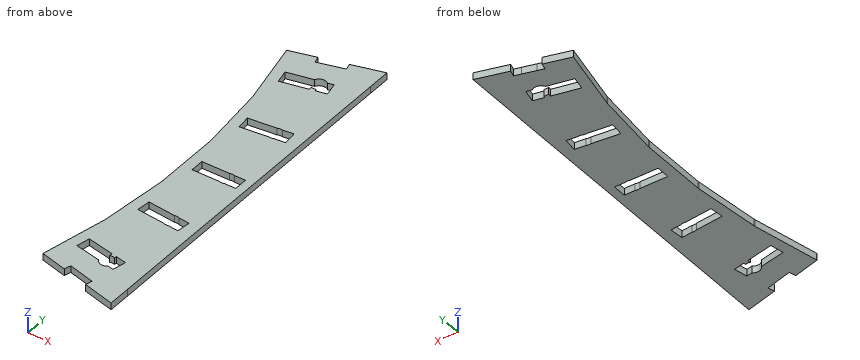
Autodesk Inventor part; units mm, degrees
ref_plane "Work Plane2" through (388.0538, -686.9281, 216.8066) normal (0, 0, 1) x (-0.9917, -0.1283, 0)
ref_plane "YZ Plane" through (0, 0, 0) normal (1, 0, 0) x (0, 1, 0)
ref_plane "XZ Plane" through (0, 0, 0) normal (0, 1, 0) x (-1, 0, 0)
ref_plane "Work Plane2" through (388.0538, -686.9281, 216.8066) normal (0, 0, 1) x (-0.9917, -0.1283, 0)
sketch "Sketch3" plane through (388.0538, -686.9281, 216.8066) normal (0, 0, 1) x (-0.9917, -0.1283, 0)
  line L0 (4.3583, 15.8159) -> (10.8533, 46.3726) construction
  line L1 (1.0044, -15.8113) -> (4.2698, 15.2569) construction
  line L2 (1.0044, -15.8113) -> (4.2698, 15.2569) construction
  line L3 (0.9748, -47.6157) -> (0.9748, -16.3764) construction
  line L4 (0.9748, -47.6157) -> (0.9748, -16.3764) construction
  line L5 (4.2698, -79.2491) -> (1.0044, -48.1809) construction
  line L6 (4.2698, -79.2491) -> (1.0044, -48.1809) construction
  line L7 (10.9998, 46.9192) -> (20.6533, 76.6296) construction
  line L8 (4.3583, 15.8159) -> (10.8533, 46.3726) construction
  line L9 (10.9998, 46.9192) -> (20.6533, 76.6296) construction
  line L10 (20.6533, 76.6296) -> (-103.8397, 124.4179) construction
  line L11 (-117.8064, 81.4327) -> (10.9998, 46.9192) construction
  line L12 (10.8533, 46.3726) -> (-117.9529, 80.8861) construction
  line L13 (-127.3499, 36.6764) -> (4.3583, 15.8159) construction
  line L14 (4.2698, 15.2569) -> (-127.4385, 36.1175) construction
  line L15 (0.9748, -16.3764) -> (-132.1925, -9.3974) construction
  line L16 (-132.1629, -8.8323) -> (1.0044, -15.8113) construction
  line L17 (1.0044, -48.1809) -> (-132.1629, -55.1599) construction
  line L18 (-132.1925, -54.5947) -> (0.9748, -47.6157) construction
  line L19 (-127.4385, -100.1096) -> (4.2698, -79.2491) construction
  line L20 (19.0965, 77.2271) -> (9.3891, 47.3508)
  line L21 (9.3891, 47.3508) -> (9.2426, 46.8041)
  line L22 (9.2426, 46.8041) -> (2.7113, 16.0767)
  line L23 (2.7113, 16.0767) -> (2.6228, 15.5178)
  line L24 (2.6228, 15.5178) -> (-0.6609, -15.724)
  line L25 (-0.6609, -15.724) -> (-0.6905, -16.2891)
  line L26 (-0.6905, -16.2891) -> (-0.6905, -47.703)
  line L27 (-0.6905, -47.703) -> (-0.6609, -48.2681)
  line L28 (-0.6609, -48.2681) -> (2.6228, -79.5099)
  line L29 (2.6228, -79.5099) -> (-36.3059, -75.4184)
  line L30 (-36.3059, -75.4184) -> (-19.8322, 81.3187)
  line L31 (-19.8322, 81.3187) -> (19.0965, 77.2271)
  line L32 (-127.4385, 36.1175) -> (-129.1369, 19.9578) construction
  point P0 (296.7492, -731.0239)
  dimension "d32" = 1.6652
  dimension "d33" = 1.6652
  dimension "d34" = 1.6652
  dimension "d35" = 1.6652
  dimension "d36" = 1.6652
  dimension "d37" = 29.21
extrude "Extrusion3" add sketch "Sketch3" along normal blind 3.175
sketch "Sketch5" plane through (388.0538, -686.9281, 219.9816) normal (0, 0, 1) x (0.9917, 0.1283, 0)
  line L0 (-19.0965, -77.2271) -> (19.8322, -81.3187)
  line L1 (-19.0965, -77.2271) -> (-19.1979, -77.4913)
  line L2 (-19.1979, -77.4913) -> (-7.3415, -82.0426)
  line L3 (4.515, -86.5938) -> (18.7052, -92.0409)
  line L4 (19.8322, -81.3187) -> (36.3059, 75.4184)
  line L5 (19.8322, -81.3187) -> (18.7052, -92.0409)
  line L6 (-18.0601, -74.5272) -> (-19.1979, -77.4913) construction
  line L7 (36.3059, 75.4184) -> (37.4328, 86.1406)
  line L8 (37.4328, 86.1406) -> (22.4202, 83.7628)
  line L9 (9.8766, 81.7761) -> (-2.6671, 79.7894)
  line L10 (36.3059, 75.4184) -> (-2.6228, 79.5099)
  line L11 (-2.6671, 79.7894) -> (-2.6228, 79.5099)
  line L12 (-2.6671, 79.7894) -> (-2.1704, 76.6535) construction
  line L13 (1.5509, -85.456) -> (-4.3773, -83.1804)
  line L14 (2.6887, -82.4919) -> (1.5509, -85.456)
  line L15 (-3.2395, -80.2163) -> (2.6887, -82.4919)
  line L16 (-3.2395, -80.2163) -> (-4.3773, -83.1804)
  line L17 (19.781, 80.1302) -> (13.5092, 79.1369)
  line L18 (19.2843, 83.2662) -> (19.781, 80.1302)
  line L19 (13.0125, 82.2728) -> (19.2843, 83.2662)
  line L20 (13.0125, 82.2728) -> (13.5092, 79.1369)
  line L21 (-4.3773, -83.1804) -> (-7.3415, -82.0426)
  line L22 (-3.2395, -80.2163) -> (-4.3773, -83.1804)
  line L23 (-6.2036, -79.0785) -> (-3.2395, -80.2163)
  line L24 (-7.3415, -82.0426) -> (-6.2036, -79.0785)
  line L25 (4.515, -86.5938) -> (1.5509, -85.456)
  line L26 (5.6528, -83.6297) -> (4.515, -86.5938)
  line L27 (2.6887, -82.4919) -> (5.6528, -83.6297)
  line L28 (2.6887, -82.4919) -> (1.5509, -85.456)
  line L29 (22.9169, 80.6269) -> (19.781, 80.1302)
  line L30 (22.4202, 83.7628) -> (22.9169, 80.6269)
  line L31 (19.2843, 83.2662) -> (22.4202, 83.7628)
  line L32 (19.2843, 83.2662) -> (19.781, 80.1302)
  line L33 (13.5092, 79.1369) -> (10.3733, 78.6402)
  line L34 (13.0125, 82.2728) -> (13.5092, 79.1369)
  line L35 (9.8766, 81.7761) -> (13.0125, 82.2728)
  line L36 (10.3733, 78.6402) -> (9.8766, 81.7761)
  point P0 (-296.7492, 731.0239)
  point P1 (19.781, 80.1302)
  point P2 (13.5092, 79.1369)
  point P3 (2.6887, -82.4919)
extrude "Extrusion4" add sketch "Sketch5" against normal blind 3.175 contours L10 L11 L9 L36 L33 L17 L29 L30 L8 L7 | L0 L5 L3 L26 L27 L15 L23 L24 L2 L1
sketch "Sketch6" plane through (388.0538, -686.9281, 219.9816) normal (0, 0, 1) x (0.9917, 0.1283, 0)
  line L0 (16.6451, 79.6336) -> (18.6318, 67.0899) construction
  line L1 (-0.2754, -81.3541) -> (4.2759, -69.4976) construction
  line L2 (18.7052, -92.0409) -> (37.4328, 86.1406) construction
  line L3 (28.069, -2.9502) -> (17.9647, -1.8882) construction
  line L4 (-6.2036, -79.0785) -> (5.6528, -83.6297) construction
  line L5 (22.9169, 80.6269) -> (10.3733, 78.6402) construction
  point P0 (-296.7492, 731.0239)
  dimension "d23" = 12.7
  dimension "d24" = 12.7
  dimension "d55" = 10.16
hole "Hole2" at (401.2076, -755.3034, 219.9816) at (397.9274, -618.0027, 219.9816) at (406.1123, -686.4967, 219.9816) direction (0, 0, -1) diameter 6.7564 depth 13.6144
sketch "Sketch7" plane through (388.0538, -686.9281, 219.9816) normal (0, 0, 1) x (0.9917, 0.1283, 0)
  line L0 (0.6609, 15.724) -> (-2.6228, -15.5178) construction
  line L1 (-0.981, 0.1031) -> (10.3864, -1.0917) construction
  line L2 (3.6239, -3.5734) -> (16.4852, -4.9251)
  line L3 (16.4852, -4.9251) -> (17.1489, 1.3901)
  line L4 (17.1489, 1.3901) -> (4.2877, 2.7418)
  line L5 (4.2877, 2.7418) -> (3.6239, -3.5734)
  line L6 (3.6239, -3.5734) -> (17.1489, 1.3901) construction
  line L7 (16.4852, -4.9251) -> (4.2877, 2.7418) construction
  circle A0 centre (17.9647, -1.8882) radius 3.3782 construction
  line L8 (10.8679, -38.2669) -> (-1.7816, -35.5781)
  line L9 (-1.7816, -35.5781) -> (-0.4614, -29.3669)
  line L10 (-0.4614, -29.3669) -> (12.1881, -32.0556)
  line L11 (12.1881, -32.0556) -> (10.8679, -38.2669)
  line L12 (10.8679, -38.2669) -> (-0.4614, -29.3669) construction
  line L13 (-1.7816, -35.5781) -> (12.1881, -32.0556) construction
  line L14 (-10.5029, -66.8425) -> (1.7962, -70.8387)
  line L15 (1.7962, -70.8387) -> (3.7585, -64.7995)
  line L16 (3.7585, -64.7995) -> (-8.5407, -60.8033)
  line L17 (-8.5407, -60.8033) -> (-10.5029, -66.8425)
  line L18 (-10.5029, -66.8425) -> (3.7585, -64.7995) construction
  line L19 (1.7962, -70.8387) -> (-8.5407, -60.8033) construction
  line L20 (18.5865, 35.1711) -> (5.6544, 35.1711)
  line L21 (5.6544, 35.1711) -> (5.6544, 28.8211)
  line L22 (5.6544, 28.8211) -> (18.5865, 28.8211)
  line L23 (18.5865, 28.8211) -> (18.5865, 35.1711)
  line L24 (18.5865, 35.1711) -> (5.6544, 28.8211) construction
  line L25 (5.6544, 35.1711) -> (18.5865, 28.8211) construction
  line L26 (3.6239, 67.5655) -> (4.2877, 61.2503)
  line L27 (4.2877, 61.2503) -> (17.1489, 62.6021)
  line L28 (17.1489, 62.6021) -> (16.4852, 68.9173)
  line L29 (16.4852, 68.9173) -> (3.6239, 67.5655)
  line L30 (3.6239, 67.5655) -> (17.1489, 62.6021) construction
  line L31 (4.2877, 61.2503) -> (16.4852, 68.9173) construction
  line L32 (-9.3891, -47.3508) -> (-19.0965, -77.2271) construction
  line L33 (-14.2428, -62.289) -> (-3.3722, -65.821) construction
  line L34 (-2.7113, -16.0767) -> (-9.2426, -46.8041) construction
  line L35 (-5.977, -31.4404) -> (5.2033, -33.8169) construction
  line L36 (0.6905, 47.703) -> (0.6905, 16.2891) construction
  line L37 (0.6905, 31.9961) -> (12.1205, 31.9961) construction
  line L38 (-2.6228, 79.5099) -> (0.6609, 48.2681) construction
  line L39 (-0.981, 63.889) -> (10.3864, 65.0838) construction
  line L40 (18.7804, -5.1664) -> (19.4442, 1.1488)
  line L41 (19.4442, 1.1488) -> (24.4964, 0.6178)
  line L42 (24.4964, 0.6178) -> (23.8326, -5.6974)
  line L43 (23.8326, -5.6974) -> (18.7804, -5.1664)
  line L44 (18.7804, -5.1664) -> (24.4964, 0.6178) construction
  line L45 (19.4442, 1.1488) -> (23.8326, -5.6974) construction
  line L46 (13.1254, -38.7467) -> (14.4456, -32.5355)
  line L47 (14.4456, -32.5355) -> (19.4146, -33.5916)
  line L48 (19.4146, -33.5916) -> (18.0943, -39.8029)
  line L49 (18.0943, -39.8029) -> (13.1254, -38.7467)
  line L50 (13.1254, -38.7467) -> (19.4146, -33.5916) construction
  line L51 (14.4456, -32.5355) -> (18.0943, -39.8029) construction
  line L52 (20.8944, 28.8211) -> (20.8944, 35.1711)
  line L53 (20.8944, 35.1711) -> (25.9744, 35.1711)
  line L54 (25.9744, 35.1711) -> (25.9744, 28.8211)
  line L55 (25.9744, 28.8211) -> (20.8944, 28.8211)
  line L56 (20.8944, 28.8211) -> (25.9744, 35.1711) construction
  line L57 (20.8944, 35.1711) -> (25.9744, 28.8211) construction
  line L58 (3.9912, -71.5519) -> (5.9534, -65.5127)
  line L59 (5.9534, -65.5127) -> (10.7848, -67.0825)
  line L60 (10.7848, -67.0825) -> (8.8225, -73.1217)
  line L61 (8.8225, -73.1217) -> (3.9912, -71.5519)
  line L62 (3.9912, -71.5519) -> (10.7848, -67.0825) construction
  line L63 (5.9534, -65.5127) -> (8.8225, -73.1217) construction
  line L64 (19.4442, 62.8433) -> (18.7804, 69.1585)
  line L65 (18.7804, 69.1585) -> (23.8326, 69.6895)
  line L66 (23.8326, 69.6895) -> (24.4964, 63.3743)
  line L67 (24.4964, 63.3743) -> (19.4442, 62.8433)
  line L68 (19.4442, 62.8433) -> (23.8326, 69.6895) construction
  line L69 (18.7804, 69.1585) -> (24.4964, 63.3743) construction
  point P0 (-296.7492, 731.0239)
  point P1 (5.2033, -33.8169)
  point P2 (-3.3722, -65.821)
  point P3 (12.1205, 31.9961)
  point P4 (10.3864, 65.0838)
  point P5 (21.6384, -2.2743)
  dimension "d38" = 11.43
  dimension "d39" = 6.35
  dimension "d40" = 12.9321
  dimension "d41" = 11.43
  dimension "d42" = 11.43
  dimension "d43" = 11.43
  dimension "d44" = 11.43
  dimension "d45" = 6.35
  dimension "d46" = 6.35
  dimension "d47" = 6.35
  dimension "d48" = 6.35
  dimension "d49" = 12.9321
  dimension "d50" = 12.9321
  dimension "d51" = 12.9321
  dimension "d52" = 12.9321
  dimension "d66" = 6.35
  dimension "d67" = 5.08
  dimension "d68" = 2.3079
  dimension "d69" = 6.35
  dimension "d70" = 5.08
  dimension "d71" = 6.35
  dimension "d72" = 5.08
  dimension "d73" = 6.35
  dimension "d74" = 5.08
  dimension "d75" = 6.35
  dimension "d76" = 5.08
  dimension "d77" = 2.3079
  dimension "d78" = 2.3079
  dimension "d79" = 2.3079
  dimension "d80" = 2.3079
extrude "Extrusion5" cut sketch "Sketch7" against normal blind 3.175
sketch "Sketch8" plane through (388.0538, -686.9281, 219.9816) normal (0, 0, 1) x (0.9917, 0.1283, 0)
  line L0 (0.6609, 15.724) -> (-2.6228, -15.5178) construction
  arc A0 (16.4852, -4.9251) -> (17.1489, 1.3901) centre (17.9647, -1.8882) ccw construction
  line L1 (18.5865, 35.1711) -> (18.5865, 28.8211) construction
  line L2 (18.5865, 31.9961) -> (19.7405, 31.9961) construction
  line L3 (0.6905, 47.703) -> (0.6905, 16.2891) construction
  line L4 (10.8679, -38.2669) -> (12.1881, -32.0556) construction
  line L5 (11.528, -35.1612) -> (12.6567, -35.4012) construction
  line L6 (-2.7113, -16.0767) -> (-9.2426, -46.8041) construction
  point P0 (-296.7492, 731.0239)
  point P1 (-0.6491, 3.2607)
  point P2 (0.6905, 35.1711)
  point P3 (-5.3169, -28.3348)
  dimension "d56" = 19.05
  dimension "d57" = 19.05
  dimension "d58" = 19.05
hole "Hole3" at (403.5277, -652.6645, 219.9816) at (405.1463, -720.4137, 219.9816) direction (0, 0, -1) diameter 6.7564 depth 13.6144
equation "\"d33\" = d32"
equation "\"d34\" = d32"
equation "\"d36\" = d32"
equation "\"d41\" = d38"
equation "\"d42\" = d38"
equation "\"d43\" = d38"
equation "\"d44\" = d38"
equation "\"d45\" = d39"
equation "\"d46\" = d39"
equation "\"d47\" = d39"
equation "\"d48\" = d39"
equation "\"d49\" = d40"
equation "\"d50\" = d40"
equation "\"d51\" = d40"
equation "\"d52\" = d40"
equation "\"d57\" = d56"
properties part number "Back Plate" material "Aluminum 6061"
For this review, take the finished solid that the model builds, in its own axes (mm). Give positions to 0.01 mm unless a question says otherwise; leave off trailing zeros. Order: outer loops, then holes, each group sorted by start corner. A loop starts at its lowest first (then second) coordinate and runs counter-clockwise, first axis right, second up.
1) Wall thickness on line 1 (Y direction, x = 410.5, z = 219.3); line 2 (Y direction, x = 398, z = 217); line 3 (Y direction, x = 407.5, z = 219.55): over which ranges is each line inside the solid? List them lowest first.
2) Take a section at C-C (y = -705). Give the boundary of the cut face in (x, z), then the cut area to 3 significant figures.
3) Take a section at A-A (z = 217.5). State how many separate pieces and enclosed holes the cut face has, then the cut area to 3 significant figures.
4) Take a section at B-B (y = -644). Give the boundary of the cut face in (x, z), then the cut area to 3 significant figures.
5) Insertion check: pin 1 (1.5 mm diameter, centred on x = 406.5, z = 218.5, fed in from -Y); pin 2 (1 mm diameter, centred on x = 380, z = 218.5, fed in from -Y). Each pin has a flat end and moves straight along its axis. Give the tip position at first contact, or say it passes through.
Derived:
1. line 1: y = -773.89 to -724.03, -717.66 to -689.57, -683.21 to -597.76
1. line 2: y = -767.59 to -756.78, -750.32 to -723.02, -716.65 to -689.87, -683.51 to -656.58, -650.18 to -621.38, -614.63 to -604.74
1. line 3: y = -773.16 to -723.79, -717.42 to -689.64, -683.29 to -655.35, -648.95 to -598.64
2. outline: (387.28, 216.81) - (416.72, 216.81) - (416.72, 219.98) - (387.28, 219.98) - close
2. area: 93.5 mm2
3. separate pieces: 1
3. enclosed holes: 5
3. area: 4,820 mm2
4. outline: (383.2, 216.81) - (415.26, 216.81) - (415.26, 219.98) - (383.2, 219.98) - close
4. area: 102 mm2
5. pin 1: stops at y = -773.1
5. pin 2: stops at y = -766.62
